```python
from build123d import *
from build123d.topology import SkipClean

# Parameters (mm, degrees)
SKETCH_1_R          = 5
SKETCH_1_R_2        = 4
EXTRUDE_1_DEPTH     = 25
SKETCH_3_R          = 7.5
EXTRUDE_2_DEPTH     = 10
SKETCH_4_R          = 10
EXTRUDE_3_DEPTH     = 13
SKETCH_6_R          = 5
CUT_EXTRUDE_1_DEPTH = 28


with BuildPart() as part:
    # Эскиз1 → Бобышка-Вытянуть1 (new body)
    with BuildSketch(Plane(origin=(0, 0, 0), x_dir=(1, 0, 0), z_dir=(0, 1, 0))):
        with Locations(Location((0, 0, 0), (0, 0, 270))):
            Circle(SKETCH_1_R)
        with Locations(Location((0, 0, 0), (0, 0, 270))):
            Circle(SKETCH_1_R_2, mode=Mode.SUBTRACT)
    extrude(amount=EXTRUDE_1_DEPTH)

    # Эскиз2 → Повернуть1 (revolve)
    with BuildSketch(Plane.XY, mode=Mode.PRIVATE) as revolve_1_sk:
        with BuildLine():
            Line((0, 25), (0, 40))
            ThreePointArc((0, 40), (5.303300859, 37.803300859), (7.5, 32.5))
            Line((7.5, 32.5), (7.5, 25))
            Line((7.5, 25), (0, 25))
        make_face()
    revolve(revolve_1_sk.sketch.rotate(Axis((0, 25, 0), (0, 1, 0)), 90), axis=Axis((0, 25, 0), (0, 1, 0)))

    # Эскиз3 → Бобышка-Вытянуть2 (add)
    with SkipClean():  # the faces are left unmerged after this step: merging them gives an invalid solid
        with BuildSketch(Plane.XY):
            with Locations((0, 32.5)):
                Circle(SKETCH_3_R)
        extrude(amount=EXTRUDE_2_DEPTH)

    # Эскиз4 → Бобышка-Вытянуть3 (add)
    with SkipClean():  # the faces are left unmerged after this step: merging them gives an invalid solid
        with BuildSketch(Plane.XY.offset(10)):
            with Locations(Location((0, 32.5, 0), (0, 0, 180))):
                Circle(SKETCH_4_R)
        extrude(amount=EXTRUDE_3_DEPTH)

    # Эскиз5 → Повернуть3 (revolve)
    with SkipClean():  # the faces are left unmerged after this step: merging them gives an invalid solid
        with BuildSketch(Plane(origin=(0, 0, 0), x_dir=(0, 0, -1), z_dir=(1, 0, 0)), mode=Mode.PRIVATE) as revolve_3_sk:
            Polygon((-26.75, 24.5), (-26.75, 26.5), (-25.75, 26.5), (-25.75, 23.75), (-25, 23), (-23.75, 23), (-23.75, 23.5), (-23, 23.5), (-23, 28.5), (-27.75, 28.5), (-27.75, 24.5), align=None)
        revolve(revolve_3_sk.sketch.rotate(Axis((0, 32.5, 23), (0, 0, 1)), 270), axis=Axis((0, 32.5, 23), (0, 0, 1)))

    # Эскиз6 → Вырез-Вытянуть1 (cut)
    with SkipClean():  # the faces are left unmerged after this step: merging them gives an invalid solid
        with BuildSketch(Plane.XY.offset(27.75)):
            with Locations((0, 32.5)):
                Circle(SKETCH_6_R)
        extrude(amount=-CUT_EXTRUDE_1_DEPTH, mode=Mode.SUBTRACT)


solid = part.part
```
Source: CAD feature listing. Evaluate the final solid. Frame: model axes, mm. A direction names the side the tool comes from. Give positions to 0.01 mm unless a question says otherwise; leave off trailing zeros. Loops run counter-clockwise (first coordinate to the right, second up) from the corner with the lowest first, then second, coordinate; pieces in that order, holes last. Notation, with made-up numbers: (50.25, -0.5) - (98.25, -0.5) arc R16 ccw to (98.25, 9.5) - close; hole circle Ø9 at (4, 75.5). An arc over 180 degrees is marked (long way). Use CSV: the item, a comma, the result in double quotes.
1) Cut plane C-C (z = 17). Output: boundary loops of the cut face in (x, y).
Worked out:
outline,"circle Ø20 at (0, 32.5); hole circle Ø10 at (0, 32.5)"
2) Cut plane B-B (y = 3.5). Output: boundary loops of the cut face in (x, z), and give its area (3 significant figures).
Worked out:
outline,"circle Ø10 at (0, 0); hole circle Ø8 at (0, 0)"
area,"28.3 mm^2"
3) Line query: line 1 (Y direction, x = 0, z = 13.75); line 2 (X direction, y = 11.25, z = 0); line 3 (Z direction, x = 6, y = 40). Output: solid intervals per line, ascending.
Worked out:
line 1,"y = 22.5 to 27.5, 37.5 to 42.5"
line 2,"x = -5 to -4, 4 to 5"
line 3,"z = 10 to 23"
4) Mould query, pull axis Y, two halves, no side actions, for faces 4 (the cylindrical face through (2.688, 36.716, 13.946)), 5 (the cylindrical face through (1.24, 23.08, 24.37)), 6 (the flat face through (5, 25, -2)), 7 (the flat face through (-4, 36, 27.75)). Classes: +Y half, -Y half, draft (parallel to the pull), parting line (faces both ways), or undercut.
Worked out:
face 4,"undercut"
face 5,"parting line"
face 6,"-Y half"
face 7,"draft"
5) Pin query (flat end, axial travel): P1, Ø8, axis at x = 0.5, z = 0, coming from the +Y side; P2, Ø8, axis at x = -6.5, y = 34.5, coming from the -Z side; P3, Ø6, axis at y = 13, z = 6.5, coming from the +X side. Return the tip coordinate at first contact, or that it passes through.
Worked out:
P1,"stops at y = 40"
P2,"stops at z = -6.96"
P3,"stops at x = 3.57"
6) Cut plane A-A (z = -3). Output: boundary loops of the cut face in (x, y), and give its area (3 significant figures).
Worked out:
outline,"(-6.87, 25) - (-4, 25) - (-4, 0) - (-2.65, 0) - (-2.65, 25) - (2.65, 25) - (2.65, 0) - (4, 0) - (4, 25) - (6.87, 25) - (6.87, 32.5) arc R6.87 ccw to (-6.87, 32.5) - close"
area,"245 mm^2"
7) Set-up query: faces 1 (the flat face through (0, 25, 0)), 2 (the cylindrical face through (1.041, 24.568, 27.243)), 3 (the flat face through (-3, 27, 26.75)). Return all of +Z, -Z, +X, -X, +Y, -Y with unobstructed straight access to the full face (end or side cutting, diameter ignored); none if empty.
Worked out:
face 1,"-Y"
face 2,"+Z"
face 3,"none"
